Answer from the drawing. Dimensions are ordinates in mm from the lowest x, y and z of the part. A direction names the side the tool comes from. Give positions to 0.01 mm unless a question says otherwise; leave off trailing zeros. Order: outer loops, then holes, each group sorted by start corner. A loop starts at its lowest first (then second) coordinate and runs counter-clockwise, first axis right, second up. Notation, with made-up numbers: (17.25, -26) - (33.25, -26) arc R22 cw to (33.25, 13) - close; hole circle Ø7 at (1.25, 68.25). An arc over 180 degrees is marked (long way). Answer in a Markdown table with one row per item. Add a question column.
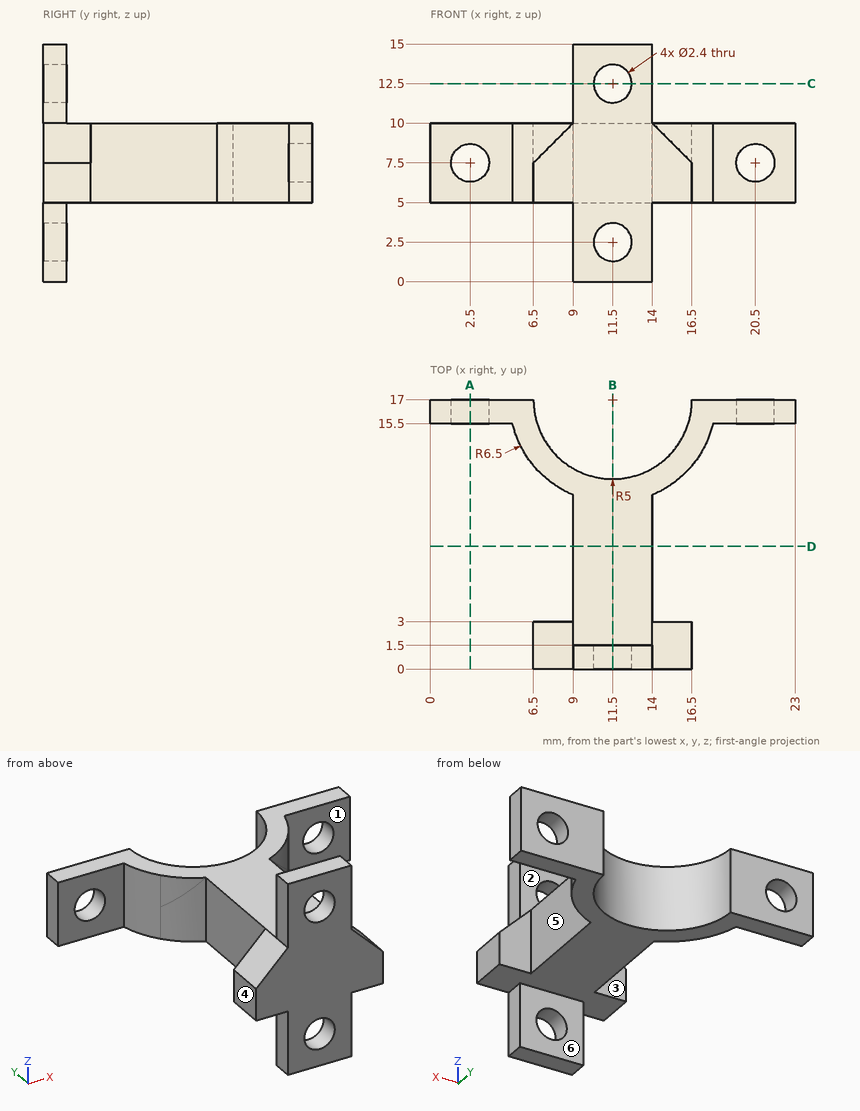
(1) Straight lines are drawn through the part: line 1 (Z direction, x = 11.5, y = 0.5); line 2 (X direction, y = 4.5, z = 5.25); line 3 (X direction, y = 0.55, z = 2.5). For each, find the intervals that lie inside material, in ascending order.
(2) For the marked faces 4, 5 and 6, determine the directions among +Z, -Z, +X, -X, +Y, -Y from which every point of the face is accessible in a straight line to the end or side of a thin tool.
(3) Find section B-B, the plane x = 11.5. Write down the section's boundary in (y, z), plus the area to 3 significant figures.
(4) Find section C-C, the plane z = 12.5. Write down the section's boundary in (x, y), plus the area to 3 significant figures.
(5) The mould has two halves that part along Y. Classify the marked faces 1, 2 and 3: +Y half, -Y half, draft (parallel to the pull), parting line (faces both ways), or undercut.
(6) Each of these flat-tipped pins is pushed along its axis until it touches: P1, Ø1.4, axis at x = 20.5, z = 7.5, coming from the -Y side; P2, Ø0.8, axis at y = 0.5, z = 11.5, coming from the +X side; P3, Ø2.5, axis at y = 6, z = 7.5, coming from the -X side; P4, Ø4, axis at x = 11.5, z = 12.5, coming from the +Y side. Where does it stop, or does it pass through?
(7) Find section A-A, the plane x = 2.5. Write down the section's boundary in (y, z).
(8) Find section D-D, the plane y = 7.75. Write down the section's boundary in (x, z), plus the area to 3 significant figures.
Answer key:
| question | item | result |
|---|---|---|
| 1 | line 1 | 0 to 1.3, 3.7 to 11.3, 13.7 to 15 |
| 1 | line 2 | 9 to 14 |
| 1 | line 3 | 9 to 10.3, 12.7 to 14 |
| 2 | face 4 | +Z, -Z, -X, -Y |
| 2 | face 5 | +Z, -Z, +X |
| 2 | face 6 | -Z, +X, -X, +Y |
| 3 | outline | (0, 0) - (1.5, 0) - (1.5, 1.3) - (0, 1.3) - close; (0, 3.7) - (1.5, 3.7) - (1.5, 5) - (12, 5) - (12, 10) - (1.5, 10) - (1.5, 11.3) - (0, 11.3) - close; (0, 13.7) - (1.5, 13.7) - (1.5, 15) - (0, 15) - close |
| 3 | area | 67.8 mm² |
| 4 | outline | (9, 0) - (10.3, 0) - (10.3, 1.5) - (9, 1.5) - close; (12.7, 0) - (14, 0) - (14, 1.5) - (12.7, 1.5) - close |
| 4 | area | 3.90 mm² |
| 5 | face 1 | -Y half |
| 5 | face 2 | +Y half |
| 5 | face 3 | undercut |
| 6 | P1 | through |
| 6 | P2 | x = 14 |
| 6 | P3 | x = 9 |
| 6 | P4 | y = 1.5 |
| 7 | outline | (15.5, 5) - (17, 5) - (17, 6.3) - (15.5, 6.3) - close; (15.5, 8.7) - (17, 8.7) - (17, 10) - (15.5, 10) - close |
| 8 | outline | (9, 5) - (14, 5) - (14, 10) - (9, 10) - close |
| 8 | area | 25.0 mm² |
